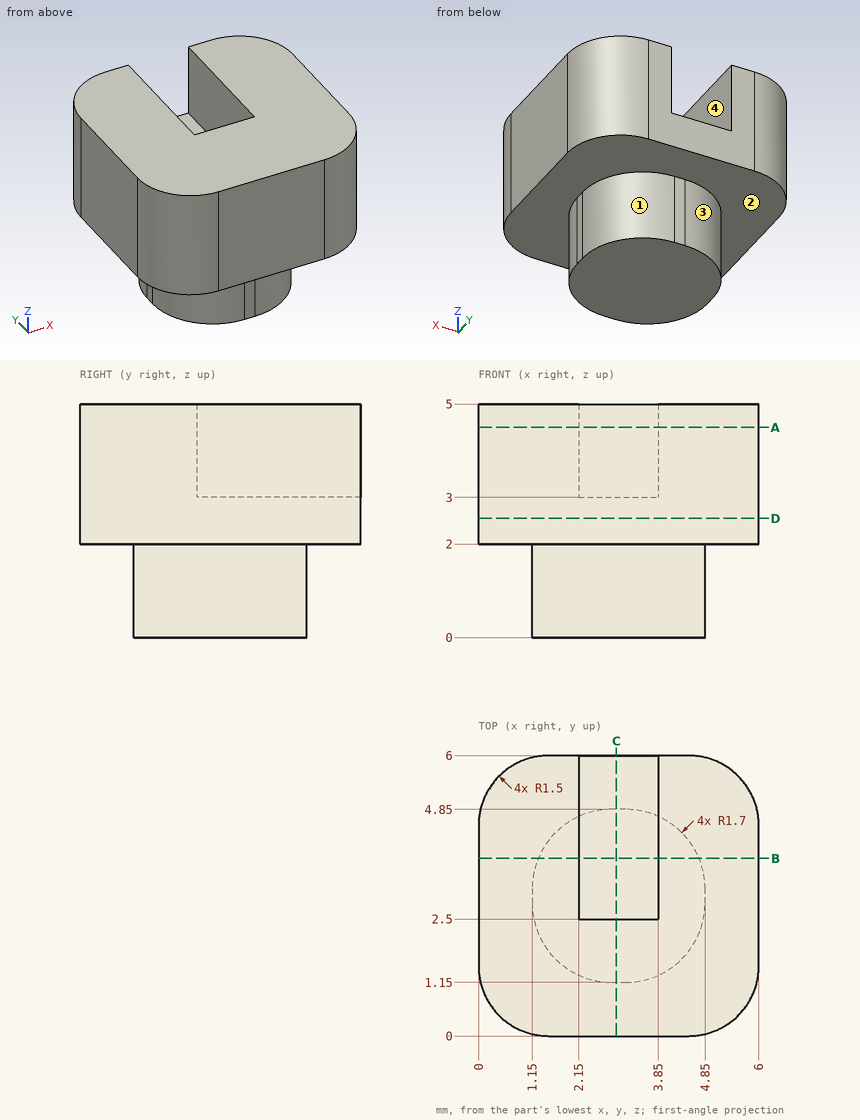
Source: three-view drawing plus pictorial views. Frame: mm from the lowest corner of the part. A direction names the side the tool comes from. Give positions to 0.01 mm unless a question says otherwise; leave off trailing zeros. Loops run counter-clockwise (first coordinate to the right, second up) from the corner with the lowest first, then second, coordinate; pieces in that order, holes last. Notation, with made-up numbers: (33.25, -38) -> (62.25, -38) arc R18 ccw to (62.25, -34) -> close; hole circle Ø7 at (-20.75, 13). An arc over 180 degrees is marked (long way). Use a Markdown table: item, result. Add a question column.
(1) Ray query, line 1 (X direction, y = 3.65, z = 3.8); line 2 (Z direction, x = 4.6, y = 5.4); line 3 (Y direction, x = 2.6, z = 4.6). Return the intervals inside material, ascending.
(2) Section query B-B (y = 3.8). Output: boundary loops of the cut face in (x, z).
(3) Section query C-C (x = 2.95). Output: boundary loops of the cut face in (y, z).
(4) Access query for the marked faces 1, 2, 3 and 4. Directions: +Z, -Z, +X, -X, +Y, -Y. A direction counts if a zero-diameter tool reaches every point of the face in a straight line with its end or side. Return the directions, or none.
(5) Section query A-A (z = 4.5). Output: boundary loops of the cut face in (x, y).
(6) Section query D-D (z = 2.55). Output: boundary loops of the cut face in (x, y).
Checked values:
| question | item | result |
|---|---|---|
| 1 | line 1 | 0 to 2.15, 3.85 to 6 |
| 1 | line 2 | 2 to 5 |
| 1 | line 3 | 0 to 2.5 |
| 2 | outline | (0, 2) -> (1.28, 2) -> (1.28, 0) -> (4.72, 0) -> (4.72, 2) -> (6, 2) -> (6, 5) -> (3.85, 5) -> (3.85, 3) -> (2.15, 3) -> (2.15, 5) -> (0, 5) -> close |
| 3 | outline | (0, 2) -> (1.15, 2) -> (1.15, 0) -> (4.85, 0) -> (4.85, 2) -> (6, 2) -> (6, 3) -> (2.5, 3) -> (2.5, 5) -> (0, 5) -> close |
| 4 | face 1 | -Z, +X, +Y |
| 4 | face 2 | -Z |
| 4 | face 3 | -Z, -X, +Y |
| 4 | face 4 | +Z, +Y |
| 5 | outline | (0, 1.5) arc R1.5 ccw to (1.5, 0) -> (4.5, 0) arc R1.5 ccw to (6, 1.5) -> (6, 4.5) arc R1.5 ccw to (4.5, 6) -> (3.85, 6) -> (3.85, 2.5) -> (2.15, 2.5) -> (2.15, 6) -> (1.5, 6) arc R1.5 ccw to (0, 4.5) -> close |
| 6 | outline | (0, 1.5) arc R1.5 ccw to (1.5, 0) -> (4.5, 0) arc R1.5 ccw to (6, 1.5) -> (6, 4.5) arc R1.5 ccw to (4.5, 6) -> (1.5, 6) arc R1.5 ccw to (0, 4.5) -> close |
